Part print with two shaded views. Sizes in mm from the minimum x, y, z corner. Round coordinates to 2 decimals unless told otherwise and drop trailing zeros. Loops run counter-clockwise (first coordinate to the right, second up) from the corner with the lowest first, then second, coordinate; pieces in that order, holes last. Notation, with made-up numbers: (-16.5, -32.5) - (34.5, -32.5) arc R18 cw to (34.5, -15.5) - close; hole circle Ø1 at (76, 42.5). An arc over 180 degrees is marked (long way). Use a Markdown table: item, result.
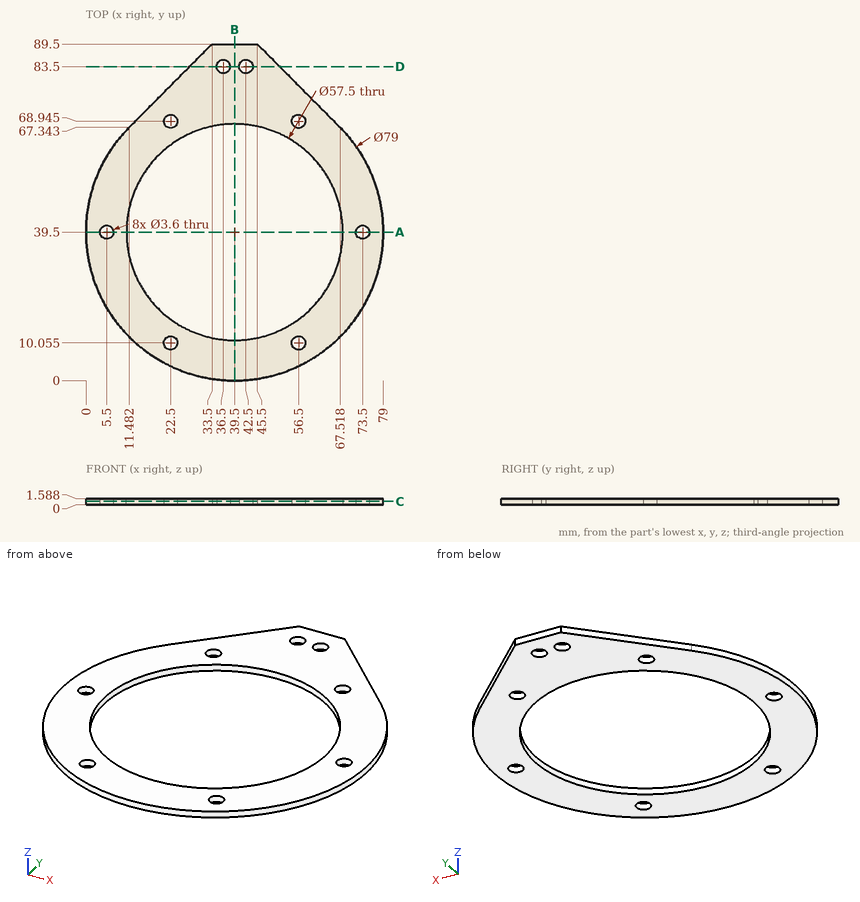
Q1. Probe line 1 (Y direction, x = 22.5, z = 0.8) (1 decimal); line 2 (Y direction, x = 39, z = 0.5) (1 decimal); line 3 (X direction, y = 82.5, z = 0.7) (1 decimal). List the from-to ranges inside material, lowest first.
Results found:
| item | result |
|---|---|
| line 1 | y = 3.8 to 8.3, 11.9 to 16.3, 62.7 to 67.1, 70.7 to 78.4 |
| line 2 | y = 0 to 10.8, 68.2 to 89.5 |
| line 3 | x = 26.5 to 35, 38 to 41, 44 to 52.5 |
Q2. Cut at D-D, the plane y = 83.5. List the corners of the cut face in (x, z).
Results found:
| item | result |
|---|---|
| outline | (27.54, 0) - (34.7, 0) - (34.7, 1.59) - (27.54, 1.59) - close; (38.3, 0) - (40.7, 0) - (40.7, 1.59) - (38.3, 1.59) - close; (44.3, 0) - (51.46, 0) - (51.46, 1.59) - (44.3, 1.59) - close |
Q3. Drop a flat-ended pin along its axis: pin 1 (3 mm diameter, centred on x = 22.5, y = 10.06, fed in from +Z). Give the stop position or say it passes through.
Results found:
| item | result |
|---|---|
| pin 1 | passes through |
Q4. Cut at C-C, the plane z = 0.9. Count the separate pieces of the cut face and the enclosed holes in it, plus the area to 3 significant figures.
Results found:
| item | result |
|---|---|
| separate pieces | 1 |
| enclosed holes | 9 |
| area | 2,530 mm2 |
Q5. Cut at B-B, the plane x = 39.5. List the corners of the cut face in (y, z).
Results found:
| item | result |
|---|---|
| outline | (0, 0) - (10.75, 0) - (10.75, 1.59) - (0, 1.59) - close; (68.25, 0) - (89.5, 0) - (89.5, 1.59) - (68.25, 1.59) - close |
Q6. Cut at A-A, the plane y = 39.5. List the corners of the cut face in (x, z).
Results found:
| item | result |
|---|---|
| outline | (0, 0) - (3.7, 0) - (3.7, 1.59) - (0, 1.59) - close; (7.3, 0) - (10.75, 0) - (10.75, 1.59) - (7.3, 1.59) - close; (68.25, 0) - (71.7, 0) - (71.7, 1.59) - (68.25, 1.59) - close; (75.3, 0) - (79, 0) - (79, 1.59) - (75.3, 1.59) - close |
